```python
from build123d import *

# Parameters (mm, degrees)
SKETCH2_W                                           = 25.4
SKETCH2_H                                           = 63.5
BOSS_EXTRUDE1_DEPTH                                 = 35.17596
SKETCH3_W                                           = 25.4
SKETCH3_H                                           = 21.05
BOSS_EXTRUDE2_DEPTH                                 = 25.4
F_1_4_0_25_DIAMETER_HOLE1_D                         = 6.35
F_1_0MM_DOWEL_HOLE1_D                               = 6.3
F_1_0MM_DOWEL_HOLE1_DEPTH                           = 8.9916
F_1_0MM_DOWEL_HOLE1_TIP                             = 1.89271095
F_4_0MM_DOWEL_HOLE1_D                               = 4
F_4_0MM_DOWEL_HOLE1_DEPTH                           = 15.24
F_4_0MM_DOWEL_HOLE1_TIP                             = 1.201721238
CBORE_FOR_10_BINDING_HEAD_MACHINE_SCREW_D           = 5.1054
CBORE_FOR_10_BINDING_HEAD_MACHINE_SCREW_DEPTH       = 35.17596
CBORE_FOR_10_BINDING_HEAD_MACHINE_SCREW_CBORE_D     = 11.1125
CBORE_FOR_10_BINDING_HEAD_MACHINE_SCREW_CBORE_DEPTH = 5.08


with BuildPart() as part:
    # Sketch2 → Boss-Extrude1 (new body)
    with BuildSketch(Plane(origin=(0, 0, 0), x_dir=(0, 0, -1), z_dir=(1, 0, 0))):
        with Locations((-225.049350785, -379.861725806)):
            Rectangle(SKETCH2_W, SKETCH2_H)
    extrude(amount=-BOSS_EXTRUDE1_DEPTH)

    # Sketch3 → Boss-Extrude2 (add)
    with BuildSketch(Plane.ZY.offset(35.17596)):
        with Locations((225.049350785, -358.636725806)):
            Rectangle(SKETCH3_W, SKETCH3_H)
    extrude(amount=BOSS_EXTRUDE2_DEPTH)

    # 1/4 (0.25) Diameter Hole1 (through all)
    with Locations(Plane(origin=(0, -348.111725806, 0), x_dir=(1, 0, 0), z_dir=(0, 1, 0))):
        with Locations((-47.87596, -225.049350785)):
            Hole(F_1_4_0_25_DIAMETER_HOLE1_D / 2)

    # Ø1.0mm Dowel Hole1
    with Locations(Plane(origin=(0, 0, 0), x_dir=(0, 0, -1), z_dir=(1, 0, 0))):
        with Locations((-231.549350785, -356.861725806), (-218.549350785, -356.861725806), (-231.549350785, -402.861725805), (-218.549350785, -402.861725805)):
            Hole(F_1_0MM_DOWEL_HOLE1_D / 2, depth=F_1_0MM_DOWEL_HOLE1_DEPTH)
            with Locations((0, 0, -(F_1_0MM_DOWEL_HOLE1_DEPTH + F_1_0MM_DOWEL_HOLE1_TIP / 2))):  # 118° drill point
                Cone(0, F_1_0MM_DOWEL_HOLE1_D / 2, F_1_0MM_DOWEL_HOLE1_TIP, mode=Mode.SUBTRACT)

    # Ø4.0mm Dowel Hole1
    with Locations(Plane(origin=(0, 0, 237.749350785), x_dir=(-1, 0, 0), z_dir=(0, 0, 1))):
        with Locations((9.83125001, 371.924225806), (9.83125001, 387.799225806)):
            Hole(F_4_0MM_DOWEL_HOLE1_D / 2, depth=F_4_0MM_DOWEL_HOLE1_DEPTH)
            with Locations((0, 0, -(F_4_0MM_DOWEL_HOLE1_DEPTH + F_4_0MM_DOWEL_HOLE1_TIP / 2))):  # 118° drill point
                Cone(0, F_4_0MM_DOWEL_HOLE1_D / 2, F_4_0MM_DOWEL_HOLE1_TIP, mode=Mode.SUBTRACT)

    # CBORE for #10 Binding Head Machine Screw1
    with Locations(Plane(origin=(0, 0, 0), x_dir=(0, 0, -1), z_dir=(1, 0, 0))):
        with Locations((-225.049350785, -381.861725806)):
            CounterBoreHole(CBORE_FOR_10_BINDING_HEAD_MACHINE_SCREW_D / 2, CBORE_FOR_10_BINDING_HEAD_MACHINE_SCREW_CBORE_D / 2, CBORE_FOR_10_BINDING_HEAD_MACHINE_SCREW_CBORE_DEPTH, depth=CBORE_FOR_10_BINDING_HEAD_MACHINE_SCREW_DEPTH)


solid = part.part
```
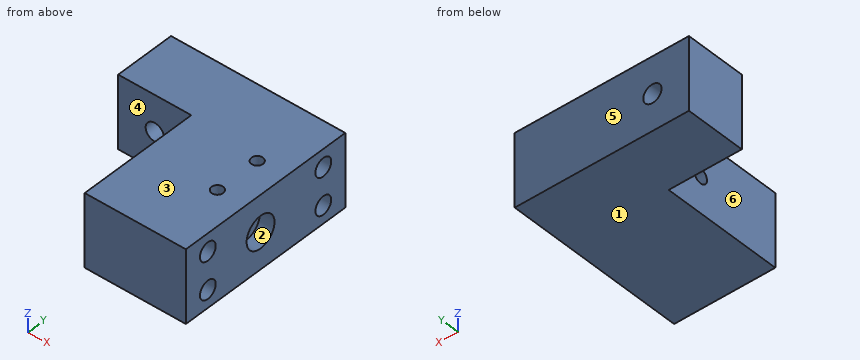
Geometry: final body of the model. Coordinates: model frame, mm. Face numbers are marked on the shaded views. A direction names the side the tool comes from. Coordinates: 2 decimals unless noted, no trailing zeros. Order: outer loops, then holes, each group sorted by start corner. A loop starts at its lowest first (then second) coordinate and runs counter-clockwise, first axis right, second up. Notation, with made-up numbers: (0.25, 51.25) -> (53.25, 51.25) arc R13 cw to (53.25, 56.25) -> close; hole circle Ø5 at (37.5, -37). An arc over 180 degrees is marked (long way). Write item = value, one per line.
(1) Access query for the marked faces 5 and 6. Directions: +Z, -Z, +X, -X, +Y, -Y. A direction counts if a zero-diameter tool reaches every point of the face in a straight line with its end or side. Return the directions, or none.
Solved:
face_5 = +Z, -Z, +X, -X, +Y
face_6 = +Z, -Z, -X, -Y
(2) Cut plane A-A on z = 223.5. Return loops of the section in (x, y).
Solved:
outline = (-60.58, -369.16) -> (-50.65, -369.16) -> (-50.65, -348.11) -> (-60.58, -348.11) -> close; (-45.1, -369.16) -> (-35.18, -369.16) -> (-35.18, -379.83) -> (-5.08, -379.83) -> (-5.08, -376.53) -> (0, -376.53) -> (0, -348.11) -> (-45.1, -348.11) -> close; (-35.18, -411.61) -> (0, -411.61) -> (0, -387.2) -> (-5.08, -387.2) -> (-5.08, -383.89) -> (-35.18, -383.89) -> close; hole circle Ø4 at (-9.83, -387.8); hole circle Ø4 at (-9.83, -371.92)
(3) Line query: line 1 (Y direction, x = -44, z = 216.5); line 2 (X direction, y = -373, z = 229.5); line 3 (X direction, y = -372.5, z = 234.5). Output: solid intervals per line, ascending.
Solved:
line_1 = -369.16 to -348.11
line_2 = -35.18 to -11.52, -8.15 to 0
line_3 = -35.18 to -11.75, -7.92 to 0
(4) Cut plane B-B on x = -6. Return loops of the section in (y, z).
Solved:
outline = (-411.61, 212.35) -> (-348.11, 212.35) -> (-348.11, 237.75) -> (-411.61, 237.75) -> close; hole circle Ø6.3 at (-402.86, 218.55); hole circle Ø6.3 at (-402.86, 231.55); hole circle Ø5.11 at (-381.86, 225.05); hole circle Ø6.3 at (-356.86, 218.55); hole circle Ø6.3 at (-356.86, 231.55)
(5) Cut plane D-D on y = -377.5. Return loops of the section in (x, z).
Solved:
outline = (-35.18, 212.35) -> (0, 212.35) -> (0, 221.61) -> (-5.08, 221.61) -> (-5.08, 228.49) -> (0, 228.49) -> (0, 237.75) -> (-35.18, 237.75) -> close
(6) Pull-direction query (Z, two-part tool) for the marked faces 1, 2, 3 and 4; classes: pulls with the +Z half, pulls with the -Z half, needs draft (parallel to the pull), parting line crosses it, or undercut.
Solved:
face_1 = pulls with the -Z half
face_2 = undercut
face_3 = pulls with the +Z half
face_4 = needs draft
(7) Cut plane C-C on y = -394. Return loops of the section in (x, z).
Solved:
outline = (-35.18, 212.35) -> (0, 212.35) -> (0, 237.75) -> (-35.18, 237.75) -> close
(8) Pin query (flat end, axial travel): pin 1 Ø6.5 at (y, z) = (-381.86, 225.05) entering from +X; pin 2 Ø1 at (x, z) = (-50, 222) entering from -Y; pin 3 Ø2 at (y, z) = (-403, 224.5) entering from -X; pin 4 Ø4 at (x, y) = (-37.5, -390.5) entering from +Z. Return the tip coordinate at first contact, or that it passes through.
Solved:
pin_1 = -5.08
pin_2 = -369.16
pin_3 = -35.18
pin_4 = through
